Input: part model. Units: mm. Frame: model coordinates. A direction names the side the tool comes from. Coordinates: 2 decimals unless noted, no trailing zeros. Order: outer loops, then holes, each group sorted by start corner. A loop starts at its lowest first (then second) coordinate and runs counter-clockwise, first axis right, second up. Notation, with made-up numbers: (-17, 63) - (-4, 63) arc R18 ccw to (-4, 69) - close; hole circle Ø8 at (1.25, 23). An arc over 180 degrees is marked (long way). Use a Markdown table: item, result. Add a question column.
Autodesk Inventor part; units mm, degrees
ref_plane "YZ Plane" through (0, 0, 0) normal (1, 0, 0) x (0, 1, 0)
ref_plane "XZ Plane" through (0, 0, 0) normal (0, 1, 0) x (-1, 0, 0)
ref_plane "XY Plane" through (0, 0, 0) normal (0, 0, 1) x (1, 0, 0)
sketch "Sketch2" plane through (0, 0, 0) normal (0, 1, 0) x (-1, 0, 0)
  line L0 (90.4875, -192.0875) -> (-61.9125, -192.0875)
  line L1 (-61.9125, -192.0875) -> (-61.9125, -249.2375)
  line L2 (-61.9125, -249.2375) -> (90.4875, -249.2375)
  line L3 (90.4875, -249.2375) -> (90.4875, -192.0875)
  dimension "d5" = 152.4
  dimension "d6" = 57.15
extrude "Plate1" add sketch "Sketch2" along normal blind 3.175
sketch "Sketch3" plane through (61.9125, 3.176, -192.0865) normal (0, 0, 1) x (1, 0, 0)
  line L0 (-152.4, 0) -> (0, 0)
  line L1 (0, 0) -> (0, 22.224)
  line L2 (0, 22.224) -> (-152.4, 22.224)
  line L3 (-152.4, 22.224) -> (-152.4, 0)
edge flange "Flange1" height 25.4 angle 90 thickness 3.175 bend radius 0 thickness toward (0, 0, 1) relief tear relief width 3.175 relief depth 1.5875 corner gap 3.175 corner form 0 edges at (-14.2875, 3.175, -192.0875) (-14.2875, 3.175, -249.2375) wall of the first edge with corners at (-90.4875, 3.176, -192.0865) (61.9125, 3.176, -192.0865) (61.9125, 25.4, -192.0865) (-90.4875, 25.4, -192.0865)
bend "Bend1"
corner "Corner1"
sketch "Sketch4" plane through (0, 3.175, 0) normal (0, 1, 0) x (1, 0, 0)
  line L0 (-14.2875, 204.7865) -> (-14.2875, 236.5365) construction
  line L1 (-90.4875, 188.9115) -> (61.9125, 188.9115) construction
  line L2 (-90.4875, 192.0875) -> (-90.4875, 249.2375) construction
  point P0 (0, 0)
  dimension "d20" = 31.75
  dimension "d21" = 15.875
  dimension "d22" = 76.2
hole "Hole1" at (-14.2875, 3.175, -204.7865) at (-14.2875, 3.175, -236.5365) direction (0, -1, 0) diameter 5.1054 end through all countersink diameter 9.779 countersink angle 82
equation "\"d10\" = BendReliefWidth"
equation "\"d11\" = BendReliefDepth"
equation "\"d12\" = MinimumRemnant"
equation "\"d13\" = BendRadius"
equation "\"d17\" = CornerReliefSize"
equation "\"d18\" = GapSize"
equation "\"d19\" = JacobiRadiusSize"
equation "\"BendRadius\" = Thickness"
equation "\"BendReliefWidth\" = Thickness"
equation "\"BendReliefDepth\" = 0.5 * Thickness"
equation "\"CornerReliefSize\" = 4 * Thickness"
equation "\"MinimumRemnant\" = 2 * Thickness"
equation "\"TransitionRadius\" = BendRadius"
equation "\"JacobiRadiusSize\" = BendRadius"
equation "\"GapSize\" = Thickness"
equation "\"d9\" = BendRadius"
properties part number "uchannel"
1) Reachability of faces 1 (the cylindrical face through (-15.354, 0.955, -251.508)), 2 (the flat face through (-13, 14, -192.086)) from +Z, -Z, +X, -X, +Y, -Y: full face, straight path, thin tool, end or side. Return the list, or none.
2) Cut plane A-A (y = 19). Return the cut outline in (x, z), and give its area (3 significant figures).
3) Pull-direction query (X, two-part tool) for faces 3 (the conical face through (-13.477, 0.655, -233.962)), 4 (the flat face through (61.912, 2, -221)), 5 (the flat face through (-13, 25.4, -191)); classes: pulls with the +X half, pulls with the -X half, needs draft (parallel to the pull), parting line crosses it, or undercut.
4) Cut plane C-C (z = -195). Return the cut outline in (x, y) (1 decimal).
5) Contact query for a flat-ended pin moving along its axis: P1, Ø6, axis at x = -9.5, z = -196, coming from the +Y side (3 decimals). Output: stop coordinate, or through.
6) Material intervals for L1, parallel to Z at x = -17.5, y = 16.75; L2, parallel to Y at x = 51.5, z = -230.5 (3 decimals); L3, parallel to Y at x = -12, z = -202, sorted ascending.
Computed:
| question | item | result |
|---|---|---|
| 1 | face 1 | -Z, +X, -X, -Y |
| 1 | face 2 | +X, -X, +Y |
| 2 | outline | (-90.49, -252.41) - (61.91, -252.41) - (61.91, -249.24) - (-90.49, -249.24) - close; (-90.49, -192.09) - (61.91, -192.09) - (61.91, -188.91) - (-90.49, -188.91) - close |
| 2 | area | 968 mm2 |
| 3 | face 3 | undercut |
| 3 | face 4 | pulls with the +X half |
| 3 | face 5 | needs draft |
| 4 | outline | (-90.5, 0) - (61.9, 0) - (61.9, 3.2) - (-90.5, 3.2) - close |
| 5 | P1 | stops at y = 3.175 |
| 6 | L1 | z = -252.41 to -249.24, -192.09 to -188.91 |
| 6 | L2 | y = 0 to 3.175 |
| 6 | L3 | y = 0 to 1.7 |
